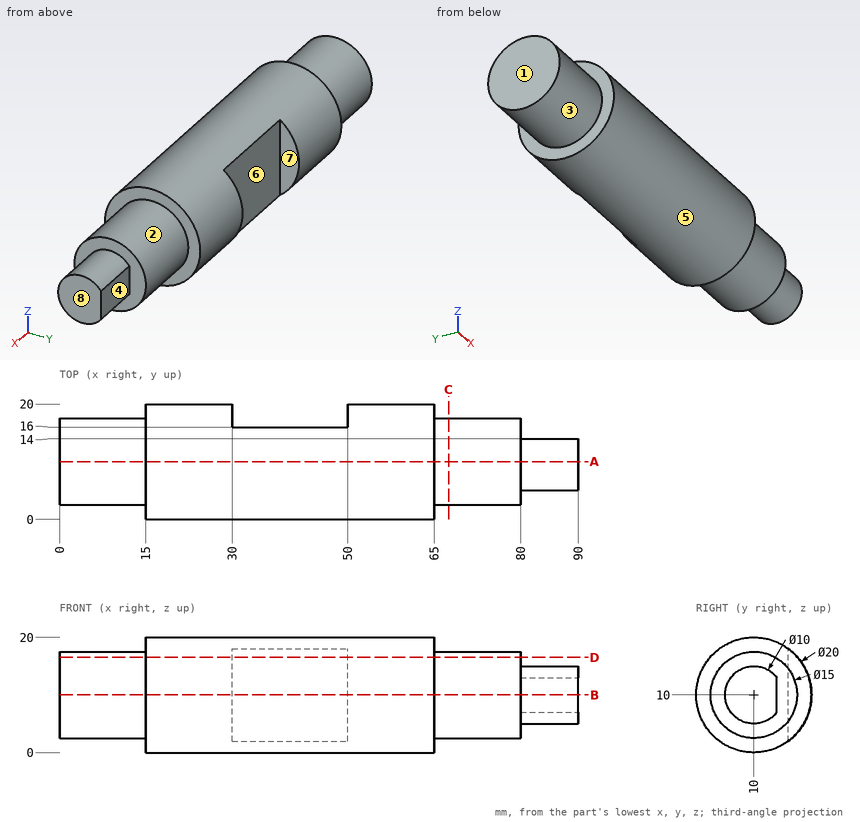
The drawing under review shows one solid part. Ordinate dimensions are in mm from its lowest x, y, z. A direction names the side the tool comes from. Give positions to 0.01 mm unless a question says otherwise; leave off trailing zeros. Loops run counter-clockwise (first coordinate to the right, second up) from the corner with the lowest first, then second, coordinate; pieces in that order, holes last. Notation, with made-up numbers: M 52,76 L 107,76 A7 cw 107,88 Z; hole C 12.25,65 d1. An arc over 180 degrees is marked long. One line per question, with ' | ' between items. Start each with the question number.
1. The part is to be moulded in two halves that separate along X. For the marked faces 5, 6, 7 and 8, say which applies: released by +X, released by -X, zero draft, split by the parting line, or undercut.
2. Add section A-A (y = 10). Write out the cut boundary in (x, z), plus the area to 3 significant figures.
3. Add section B-B (z = 10). Write out the cut boundary in (x, y), plus the area to 3 significant figures.
4. Insertion check: P1, Ø3, axis at x = 57.5, y = 2.5, coming from the -Z side; P2, Ø1.2, axis at y = 18.5, z = 10, coming from the +X side; P3, Ø5, axis at x = 49.5, y = 14, coming from the +Z side. Each pin has a flat end and moves straight along its axis. Give the tip position at first contact, or say it passes through.
5. To check wall thickness, follow L1, parallel to X at y = 17.5, z = 4.75; L2, parallel to X at y = 12.25, z = 15; L3, parallel to X at y = 15.75, z = 16.5. State the ranges of each line that lie inside material, in increasing order.
6. Add section D-D (z = 16.5). Write out the cut boundary in (x, y).
7. Add section C-C (x = 67.5). Write out the cut boundary in (y, z), plus the area to 3 significant figures.
8. For the marked faces 1, 2, 3 and 4, list the 3-axis set-ups (+Z, -Z, +X, -X, +Y, -Y) from which the entire face can be reached by the end or side of a thin tool; tool diameter is ignored.
Worked out:
1) face 5: zero draft | face 6: undercut | face 7: undercut | face 8: released by +X
2) outline: M 0,2.5 L 15,2.5 L 15,0 L 65,0 L 65,2.5 L 80,2.5 L 80,5 L 90,5 L 90,15 L 80,15 L 80,17.5 L 65,17.5 L 65,20 L 15,20 L 15,17.5 L 0,17.5 Z | area: 1,550 mm²
3) outline: M 0,2.5 L 15,2.5 L 15,0 L 65,0 L 65,2.5 L 80,2.5 L 80,5 L 90,5 L 90,14 L 80,14 L 80,17.5 L 65,17.5 L 65,20 L 50,20 L 50,16 L 30,16 L 30,20 L 15,20 L 15,17.5 L 0,17.5 Z | area: 1,460 mm²
4) P1: stops at z = 2 | P2: stops at x = 65 | P3: stops at z = 19.89
5) L1: x = 15 to 30, 50 to 65 | L2: x = 0 to 80 | L3: x = 15 to 65
6) outline: M 0,6.26 L 15,6.26 L 15,2.4 L 65,2.4 L 65,6.26 L 80,6.26 L 80,13.74 L 65,13.74 L 65,17.6 L 50,17.6 L 50,16 L 30,16 L 30,17.6 L 15,17.6 L 15,13.74 L 0,13.74 Z
7) outline: C 10,10 d15 | area: 177 mm²
8) face 1: +Z, -Z, -X, +Y, -Y | face 2: +X | face 3: -X | face 4: +Z, -Z, +X, +Y
